For this review, use the dimensioned drawing (mm, ordinates from the lowest corner) and the shaded views. A direction names the side the tool comes from. Round coordinates to 2 decimals unless told otherwise and drop trailing zeros. Write each loop counter-clockwise with the first axis right and the second up, starting at its lowest first coordinate (ties: lowest second). Pieces come first, ordered by that corner, then holes.
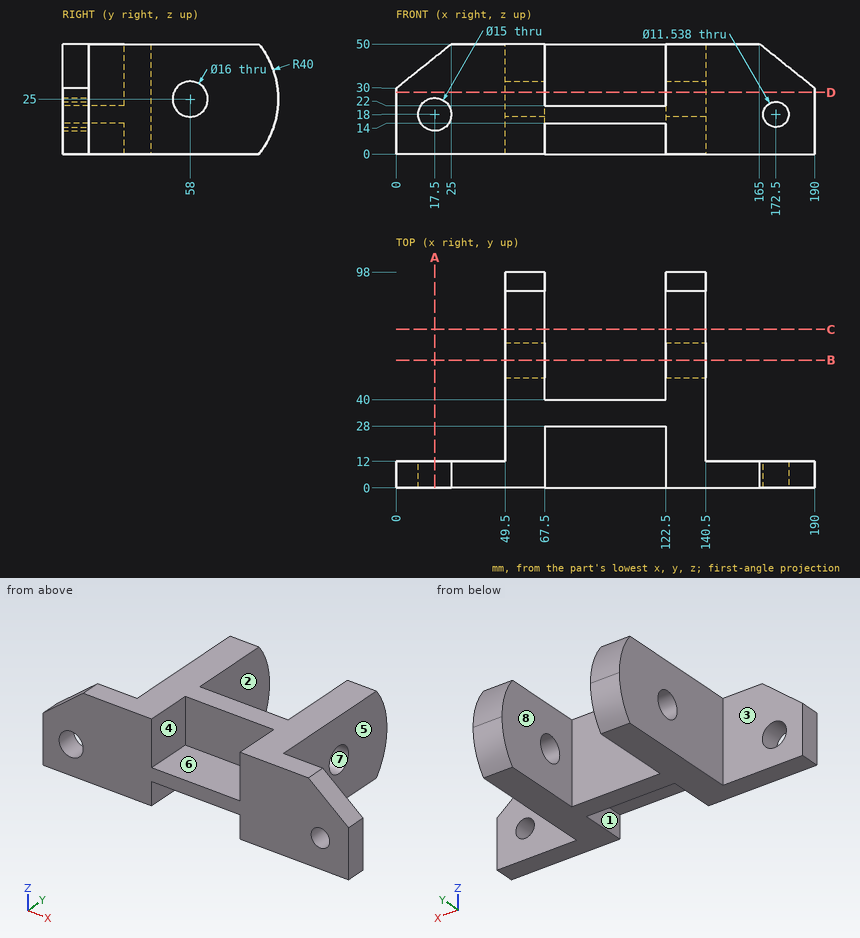
1) Add section B-B on y = 58. State the section outline as (x, z) points, and give its area (3 significant figures).
2) The part is to be moulded in two halves that separate along Z. For the marked faces 6, 7 and 8, say which applies: pulls with the +Z half, pulls with the -Z half, needs draft (parallel to the pull), parting line crosses it, or undercut.
3) For line 1 along Y through (x, z) = (53, 25); line 2 along X through (y, z) = (41.5, 32); line 3 along X through (y, z) = (6, 12), list the stretches that pass through material, from the lowest coordinate up.
4) Add section C-C on y = 72. State the section outline as (x, z) points, and give its area (3 significant figures).
5) Add section D-D on z = 28. State the section outline as (x, y) points, and give its area (3 significant figures).
6) Add section A-A on x = 17.5. State the section outline as (y, z) points, and give its area (3 significant figures).
7) For the marked faces 1, 2, 3, 4 and 5, list the 3-axis set-ups (+Z, -Z, +X, -X, +Y, -Y) from which the entire face can be reached by the end or side of a thin tool; tool diameter is ignored.
8) For P1, Ø6, axis at y = 13.5, z = 38, coming from the +X side; P2, Ø14, axis at x = 85, z = 40, coming from the -Y side; P3, Ø6, axis at y = 28.5, z = 34.5, coming from the +X side; P4, Ø8, axis at x = 116.5, y = 59, coming from the -Z side, all flat-tipped, find the tip position at first contact; note any pin that passes through.
Computed:
1. outline: (49.5, 0) - (67.5, 0) - (67.5, 17) - (49.5, 17) - close; (49.5, 33) - (67.5, 33) - (67.5, 50) - (49.5, 50) - close; (122.5, 0) - (140.5, 0) - (140.5, 17) - (122.5, 17) - close; (122.5, 33) - (140.5, 33) - (140.5, 50) - (122.5, 50) - close
1. area: 1,220 mm2
2. face 6: pulls with the +Z half
2. face 7: undercut
2. face 8: needs draft
3. line 1: y = 0 to 50, 66 to 98
3. line 2: x = 49.5 to 67.5, 122.5 to 140.5
3. line 3: x = 0 to 13, 22 to 67.5, 122.5 to 190
4. outline: (49.5, 0) - (67.5, 0) - (67.5, 50) - (49.5, 50) - close; (122.5, 0) - (140.5, 0) - (140.5, 50) - (122.5, 50) - close
4. area: 1,800 mm2
5. outline: (0, 0) - (67.5, 0) - (67.5, 28) - (122.5, 28) - (122.5, 0) - (190, 0) - (190, 12) - (140.5, 12) - (140.5, 50.58) - (122.5, 50.58) - (122.5, 40) - (67.5, 40) - (67.5, 50.58) - (49.5, 50.58) - (49.5, 12) - (0, 12) - close; (49.5, 65.42) - (67.5, 65.42) - (67.5, 97.89) - (49.5, 97.89) - close; (122.5, 65.42) - (140.5, 65.42) - (140.5, 97.89) - (122.5, 97.89) - close
5. area: 4,840 mm2
6. outline: (0, 0) - (12, 0) - (12, 10.5) - (0, 10.5) - close; (0, 25.5) - (12, 25.5) - (12, 44) - (0, 44) - close
6. area: 348 mm2
7. face 1: -Z, -Y
7. face 2: +Z, -Z, +Y
7. face 3: +Z, -Z, -X, +Y
7. face 4: +Z, -Y
7. face 5: +Z, -Z, +X, +Y
8. P1: stops at x = 183.25
8. P2: stops at y = 28
8. P3: stops at x = 140.5
8. P4: passes through
